Part model, mm, in its own coordinate system. A direction names the side the tool comes from. Round coordinates to 2 decimals unless told otherwise and drop trailing zeros. Loops run counter-clockwise (first coordinate to the right, second up) from the corner with the lowest first, then second, coordinate; pieces in that order, holes last. Notation, with made-up numbers: M 2.5,15.5 L 22.5,15.5 A6 ccw 22.5,26.5 Z; hole C 28,59 d6. An arc over 180 degrees is marked long. Put each result on its own line as item: value. Start each with the question number.
1) Pull direction X, two halves, no side cores. Call faces 3 (the flat face through (62, 0, 120)), 4 (the flat face through (59.884, 22.984, 123.708)), 5 (the flat face through (0, 20, 120)), 6 (the flat face through (109.884, 22.984, 123.708)): +X half, -X half, draft (parallel to the pull), parting line (faces both ways), or undercut.
2) Drop flat-ended pins along their axis: pin 1 Ø4 at (x, z) = (66.5, 81) entering from +Y; pin 2 Ø1.9 at (x, z) = (42, 70) entering from +Y; pin 3 Ø1.9 at (x, z) = (42, 22.5) entering from -Y. Give the stop position or say it passes through.
3) Which spindle directions (+Z, -Z, +X, -X, +Y, -Y) get a long thin tool onto all of the face, cutting with end or side? Do faces 1 (the cylindrical face through (97.21, 2.958, 237.897)), 2 (the flat face through (49.884, 22.984, 123.708)). Say none if no direction does.
4) Slice it at A-A on x = 26. Give the cut face in (y, z), then the cut area to 3 significant figures.
5) Probe line 1 along X through (y, z) = (1.9, 236); line 2 along Z through (x, y) = (51.5, 2.3); line 3 along Z through (x, y) = (96, 3.05). List the from-to ranges inside material, lowest first.
6) Slice it at B-B on z = 236. State how many separate pieces and enclosed holes the cut face has, then the cut area to 3 significant figures.
```python
from build123d import *

# Parameters (mm, degrees)
EXTRUDE_1_DEPTH       = 244
EXTRUDE_3_DEPTH       = 244
PATTERN_CURVE_1_COUNT = 11
PATTERN_CURVE_1_PITCH = 10
SKETCH_3_R            = 2.25
CUT_EXTRUDE_1_DEPTH   = 6
SKETCH_4_R            = 1.6
SKETCH_4_R_2          = 1.15
CUT_EXTRUDE_2_DEPTH   = 6


with BuildPart() as part:
    # Эскиз1 → Вытянуть1 (new body)
    with BuildSketch(Plane.XY):
        with BuildLine():
            Line((0, 40), (1.528979332, 40))
            ThreePointArc((1.528979332, 40), (2.225614441, 39.717425624), (2.528547087, 39.029399052))
            Line((2.528547087, 39.029399052), (3.5, 6))
            Line((3.5, 6), (118.5, 6))
            Line((118.5, 6), (119.471452913, 39.029399052))
            ThreePointArc((119.471452913, 39.029399052), (119.774385559, 39.717425624), (120.471020668, 40))
            Line((120.471020668, 40), (122, 40))
            Line((122, 40), (122, 0))
            Line((122, 0), (0, 0))
            Line((0, 0), (0, 40))
        make_face()
    extrude(amount=EXTRUDE_1_DEPTH)

    # Эскиз2 → Вытянуть3 (add)
    with BuildSketch(Plane.XY.offset(244)):
        with BuildLine():
            Line((10.5, 39.5), (9.25, 6))
            Line((9.25, 6), (12.75, 6))
            Line((12.75, 6), (11.5, 39.5))
            ThreePointArc((11.5, 39.5), (11, 40), (10.5, 39.5))
        make_face()
    extrude_3 = extrude(amount=-EXTRUDE_3_DEPTH)

    # Кривая1: Вытянуть3 ×11
    with Locations(*[(i * PATTERN_CURVE_1_PITCH, 0, 0) for i in range(1, PATTERN_CURVE_1_COUNT)]):
        add(extrude_3)

    # Эскиз3 → Вырез-Вытянуть1 (cut)
    with BuildSketch(Plane.XZ):
        with Locations((26, 236)):
            Circle(SKETCH_3_R)
        with Locations((96, 236)):
            Circle(SKETCH_3_R)
        with Locations(Location((96, 8, 0), (0, 0, 180))):
            Circle(SKETCH_3_R)
        with Locations(Location((26, 8, 0), (0, 0, 180))):
            Circle(SKETCH_3_R)
    extrude(amount=-CUT_EXTRUDE_1_DEPTH, mode=Mode.SUBTRACT)

    # Эскиз4 → Вырез-Вытянуть2 (cut)
    with BuildSketch(Plane(origin=(133.240090243, 0, 310.149074448), x_dir=(-1, 0, 0), z_dir=(0, -1, 0))):
        with Locations(Location((48.740090243, 89.149074448, 0), (0, 0, 180))):
            Circle(SKETCH_4_R)
        with Locations(Location((48.740090243, 229.149074448, 0), (0, 0, 180))):
            Circle(SKETCH_4_R)
        with Locations((8.990090243, 225.549074448)):
            Circle(SKETCH_4_R)
        with Locations(Location((66.510090243, 102.149074448, 0), (0, 0, 180))):
            Circle(SKETCH_4_R_2)
        with Locations(Location((81.740090243, 187.149074448, 0), (0, 0, 180))):
            Circle(SKETCH_4_R)
        with Locations(Location((91.240090243, 288.149074448, 0), (0, 0, 180))):
            Circle(SKETCH_4_R)
        with Locations(Location((91.240090243, 240.149074448, 0), (0, 0, 180))):
            Circle(SKETCH_4_R)
        with Locations(Location((25.240090243, 240.149074448, 0), (0, 0, 180))):
            Circle(SKETCH_4_R)
        with Locations(Location((25.240090243, 288.149074448, 0), (0, 0, 180))):
            Circle(SKETCH_4_R)
        with Locations(Location((81.740090243, 168.149074448, 0), (0, 0, 180))):
            Circle(SKETCH_4_R)
    extrude(amount=-CUT_EXTRUDE_2_DEPTH, mode=Mode.SUBTRACT)


solid = part.part
```
Recorded:
1. face 3: draft
1. face 4: undercut
1. face 5: -X half
1. face 6: undercut
2. pin 1: stops at y = 6
2. pin 2: stops at y = 40
2. pin 3: stops at y = 6
3. face 1: +Y, -Y
3. face 2: +Z, -Z, +Y
4. outline: M 0,0 L 6,0 L 6,5.75 L 0,5.75 Z; M 0,10.25 L 6,10.25 L 6,233.75 L 0,233.75 Z; M 0,238.25 L 6,238.25 L 6,244 L 0,244 Z
4. area: 1,410 mm2
5. line 1: x = 0 to 23.75, 28.25 to 93.75, 98.25 to 122
5. line 2: z = 0 to 121.4, 124.6 to 140.4, 143.6 to 244
5. line 3: z = 0 to 5.75, 10.25 to 233.75, 238.25 to 244
6. separate pieces: 3
6. enclosed holes: 0
6. area: 1,720 mm2
